from build123d import *

# Parameters (mm, degrees)
F0_R     = 23.414747
F1_DEPTH = 5.08
F3_DEPTH = 19.05
F4_R     = 3.876648
F5_DEPTH = 3.048


with BuildPart() as f1:
    # F0 (on Front) → F1 (new body)
    with BuildSketch(Plane.XZ):
        Circle(F0_R)
    extrude(amount=F1_DEPTH)

    # F2 (on face) → F3 (join)
    with BuildSketch(Plane.XZ.offset(5.08)):
        with BuildLine():
            ThreePointArc((8.908676, -21.653772), (0.895358, -23.397622), (-7.227794, -22.271268))
            Line((-7.227794, -22.271268), (-7.227794, -62.864996))
            ThreePointArc((-7.227794, -62.864996), (0.840441, -70.933231), (8.908676, -62.864996))
            Line((8.908676, -62.864996), (8.908676, -21.653772))
        make_face()
        with BuildLine():
            ThreePointArc((8.908676, -6.387353), (1.456869, 8.743082), (-7.227794, -5.715))
            Line((-7.227794, -5.715), (-7.227794, -22.271268))
            ThreePointArc((-7.227794, -22.271268), (0.895358, -23.397622), (8.908676, -21.653772))
            Line((8.908676, -21.653772), (8.908676, -6.387353))
        make_face()
    extrude(amount=F3_DEPTH)

    # F4 (on face) → F5 (join)
    with BuildSketch(Plane.XZ.offset(24.13)):
        with Locations((1.056986, -0.854104)):
            Circle(F4_R)
    extrude(amount=F5_DEPTH)


solid = f1.part
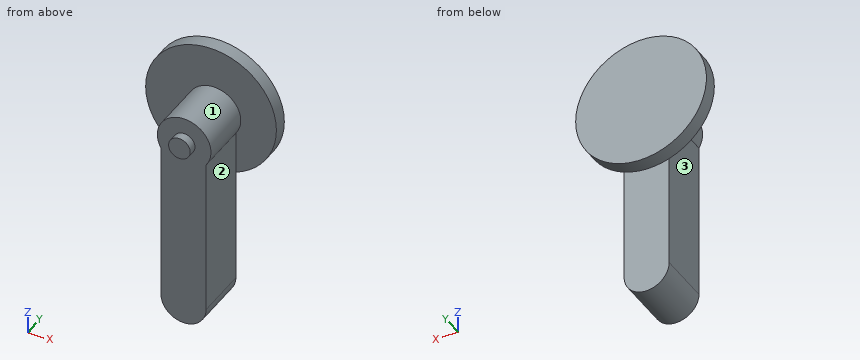
Input: part model. Units: mm. Frame: model coordinates. Face numbers are marked on the shaded views. A direction names the side the tool comes from. Give positions to 0.01 mm unless a question says otherwise; leave off trailing zeros. Loops run counter-clockwise (first coordinate to the right, second up) from the corner with the lowest first, then second, coordinate; pieces in that order, holes last. Notation, with made-up numbers: (38, 49.5) - (43, 49.5) arc R12 ccw to (43, 59.5) - close; hole circle Ø9 at (-23.75, -1). An arc over 180 degrees is marked (long way). Use CSV: the item, a comma, the result in double quotes. Start each with the question number.
Item 1: Section C-C on z = 6. Return loops of the section in (x, y).
Item 2: Section D-D on x = -16. Return loops of the section in (y, z), then the cut area to 3 significant figures.
Item 3: Line query: line 1 (Z direction, x = 1, y = -17.5); line 2 (Y direction, x = -3, z = -15); line 3 (Y direction, x = -2, z = -38). Output: solid intervals per line, ascending.
Item 4: Reachability of the marked faces 1, 2 and 3 from +Z, -Z, +X, -X, +Y, -Y: full face, straight path, thin tool, end or side. Return the list, or none.
Item 5: Contact query for flat-ended pins moving along their axis: P1, Ø21, axis at x = -2.5, z = -39.5, coming from the -Y side; P2, Ø12, axis at x = 0.5, y = -24, coming from the +Z side; P3, Ø8, axis at y = -19, z = -9, coming from the +X side; P4, Ø10, axis at x = -13, z = -60, coming from the +Y side. Output: stop coordinate, or through.
Item 6: Section A-A on x = 2. Return loops of the section in (y, z) (3 decimals).
Item 7: Section B-B on y = -16.5. Return loops of the section in (x, z) (3 decimals), then the cut area to 3 significant figures.
Ans:
1,outline,"(-22.63, -5.08) - (-5.67, -5.08) - (-5.67, -24.13) - (7.79, -24.13) - (7.79, -5.08) - (22.63, -5.08) - (22.63, 0) - (-22.63, 0) - close"
2,outline,"(-5.08, -17.1) - (0, -17.1) - (0, 17.1) - (-5.08, 17.1) - close"
2,area,"174 mm2"
3,line 1,"z = -70.93 to 8.75"
3,line 2,"y = -24.13 to 0"
3,line 3,"y = -24.13 to -5.08"
4,face 1,"-Y"
4,face 2,"-Z, +X, -Y"
4,face 3,"-Z, -X, -Y"
5,P1,"stops at y = -24.13"
5,P2,"stops at z = 8.75"
5,P3,"stops at x = 9.72"
5,P4,"passes through"
6,outline,"(-27.178, -4.614) - (-24.13, -4.614) - (-24.13, -70.849) - (-5.08, -70.849) - (-5.08, -23.329) - (0, -23.329) - (0, 23.329) - (-5.08, 23.329) - (-5.08, 8.705) - (-24.13, 8.705) - (-24.13, 2.906) - (-27.178, 2.906) - close"
7,outline,"(-7.228, -62.865) arc R8.068 ccw to (8.909, -62.865) - (8.909, -6.387) arc R9.606 ccw (long way) to (-7.228, -5.715) - close"
7,area,"1,260 mm2"
